from build123d import *

# Parameters (mm, degrees)
CYLINDER001_R     = 2
CYLINDER001_DEPTH = 4
CYLINDER002_R     = 5.25
CYLINDER002_DEPTH = 4
FILLET_R          = 2


with BuildPart() as cylinder001:
    # Cylinder001 → Cylinder001 (new body)
    with BuildSketch(Plane(origin=(0, 12, 3), x_dir=(1, 0, 0), z_dir=(0, 0, 1))):
        Circle(CYLINDER001_R)
    extrude(amount=CYLINDER001_DEPTH)


with BuildPart() as cut:
    # Cylinder002 → Cylinder002 (new body)
    with BuildSketch(Plane(origin=(0, 12, 1), x_dir=(1, 0, 0), z_dir=(0, 0, 1))):
        Circle(CYLINDER002_R)
    extrude(amount=CYLINDER002_DEPTH)

    # Fillet
    fillet_edges = [cut.edges().sort_by_distance(p)[0] for p in [
        (-5.25, 12, 5),
    ]]
    fillet(fillet_edges, radius=FILLET_R)

    # Cut: cut Cylinder001
    add(cylinder001.part, mode=Mode.SUBTRACT)


solid = cut.part
Read the model definition and answer for the solid it produces. Units are mm, in the model's axes. A direction names the side the tool comes from. Coordinates: 2 decimals unless noted, no trailing zeros. Write each loop counter-clockwise with the first axis right and the second up, starting at its lowest first coordinate (ties: lowest second). Pieces come first, ordered by that corner, then holes. Notation, with made-up numbers: (63, 87) - (99, 87) arc R9 cw to (99, 104) - close; hole circle Ø10 at (83, 40). An arc over 180 degrees is marked (long way). One line per question, with ' | ' between items.
Q1. For faces 1 (the flat face through (0, 12, 3)), 2 (the flat face through (0, 12, 1)), determine the directions among +Z, -Z, +X, -X, +Y, -Y from which every point of the face is accessible in a straight line to the end or side of a thin tool.
Result set:
face 1: +Z | face 2: -Z, +X, -X, +Y, -Y
Q2. Consider L1, parallel to Y at x = 0, z = 4.2; L2, parallel to X at y = 12.5, z = 4; L3, parallel to Y at x = 0, z = 3.85. Determine where each line is inside the solid, lowest interval first. Write a range as [from, to].
Result set:
L1: [7.15, 10], [14, 16.85] | L2: [-4.96, -1.94], [1.94, 4.96] | L3: [6.94, 10], [14, 17.06]
Q3. Find section C-C, the plane z = 3.5. Write down the section's boundary in (x, y), plus the area to 3 significant figures.
Result set:
outline: circle Ø10.37 at (0, 12); hole circle Ø4 at (0, 12) | area: 71.9 mm^2
Q4. Find section A-A, the plane x = 0. Write down the section's boundary in (y, z), plus the area to 3 significant figures.
Result set:
outline: (6.75, 1) - (17.25, 1) - (17.25, 3) arc R2 ccw to (15.25, 5) - (14, 5) - (14, 3) - (10, 3) - (10, 5) - (8.75, 5) arc R2 ccw to (6.75, 3) - close | area: 32.3 mm^2
Q5. Find section D-D, the plane z = 2.05. Write down the section's boundary in (x, y).
Result set:
outline: circle Ø10.5 at (0, 12)
Q6. Each of these flat-tipped pins is pushed along its axis until it touches: P1, Ø2.5, axis at x = 0, y = 12, coming from the +Z side; P2, Ø1, axis at x = 3.5, y = 15.5, coming from the +Z side; P3, Ø1.5, axis at x = -4, y = 14, coming from the +Z side. Where does it stop, or does it pass through?
Result set:
P1: z = 3 | P2: z = 4.6 | P3: z = 4.94
Q7. Determine the mould class of faces 3 (the cylindrical face through (0, 14, 4)), 4 (the cylindrical face through (2.82, 16.43, 1.99)), 5 (the flat face through (2, 11, 5)) for opening direction X: +X half, -X half, draft (parallel to the pull), parting line (faces both ways), or undercut.
Result set:
face 3: undercut | face 4: parting line | face 5: draft
Q8. Find section B-B, the plane y = 12. Write down the section's boundary in (x, z).
Result set:
outline: (-5.25, 1) - (5.25, 1) - (5.25, 3) arc R2 ccw to (3.25, 5) - (2, 5) - (2, 3) - (-2, 3) - (-2, 5) - (-3.25, 5) arc R2 ccw to (-5.25, 3) - close
